Input: part model. Units: mm. Frame: model coordinates. Face numbers are marked on the shaded views. A direction names the side the tool comes from. Coordinates: 2 decimals unless noted, no trailing zeros. Write each loop counter-clockwise with the first axis right and the second up, starting at its lowest first coordinate (ties: lowest second). Pieces come first, ordered by that corner, then holes. Notation, with made-up numbers: (69, -25) - (116, -25) arc R34 ccw to (116, 7) - close; hole circle Ø3 at (51, 10.25). An arc over 180 degrees is marked (long way). Use CSV: the item, a comma, the result in double quotes.
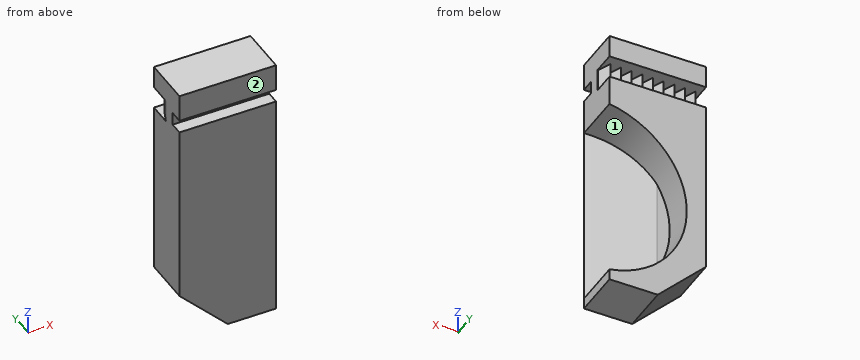
```python
from build123d import *

# Parameters (mm, degrees)
ESQUISSE2_W                = 30
ESQUISSE2_H                = 84
BOSS_EXTRU_1_DEPTH         = 15
ESQUISSE3_R                = 29
ENL_V_MAT_EXTRU_1_DEPTH    = 10
CHANFREIN1_SIZE            = 5
CHANFREIN1_SIZE_2          = 20
CHANFREIN2_SIZE            = 15
ESQUISSE7_W                = 30
ESQUISSE7_H                = 7
ENL_V_MAT_EXTRU_2_DEPTH    = 7
BOSS_EXTRU_2_DEPTH         = 7
R_P_TITION_LIN_AIRE1_COUNT = 9
R_P_TITION_LIN_AIRE1_PITCH = 3.31
ENL_V_MAT_EXTRU_3_REACH    = 56.708
ESQUISSE9_W                = 4
ESQUISSE9_H                = 4


with BuildPart() as part:
    # Esquisse2 → Boss.-Extru.1 (new body)
    with BuildSketch(Plane(origin=(0, 0, 0), x_dir=(1, 0, 0), z_dir=(0, 1, 0))):
        with Locations((-17.412854797, -1.219560319)):
            Rectangle(ESQUISSE2_W, ESQUISSE2_H)
    extrude(amount=BOSS_EXTRU_1_DEPTH)

    # Esquisse3 → Enlèv. mat.-Extru.1 (cut)
    with BuildSketch(Plane(origin=(0, 15, 0), x_dir=(1, 0, 0), z_dir=(0, 1, 0))):
        with Locations((2.587145203, 8.780439681)):
            Circle(ESQUISSE3_R)
    extrude(amount=-ENL_V_MAT_EXTRU_1_DEPTH, mode=Mode.SUBTRACT)

    # Chanfrein1
    # the kernel refuses this chamfer: 20, 5 mm, written as the material it takes off along each edge
    with BuildSketch(Plane(origin=(-2.412854797, 5, -89.288703391), x_dir=(0.14778356633657125, -0.9890197255468893, 0), z_dir=(0, 0, 1))) as chanfrein1_piece_1_section:
        Polygon((CHANFREIN1_SIZE * 0.989019725547, -CHANFREIN1_SIZE * 0.147783566337), (-CHANFREIN1_SIZE_2 * 0.147783566337, -CHANFREIN1_SIZE_2 * 0.989019725547), (0, 0), align=None)
    chanfrein1_piece_1 = extrude(amount=161.016527419, mode=Mode.PRIVATE)
    chanfrein1_piece_1 = chanfrein1_piece_1 & Plane(origin=(2.587145203, 3.276810051, -8.780439681), x_dir=(1, 0, 0), z_dir=(0, 1, 0)) * Cylinder(29, 402, mode=Mode.PRIVATE)
    add(chanfrein1_piece_1, mode=Mode.SUBTRACT)

    # Chanfrein2
    chanfrein2_edges = [part.edges().sort_by_distance(p)[0] for p in [
        (-32.412854797, 7.5, -40.780439681),
    ]]
    chamfer(chanfrein2_edges, length=CHANFREIN2_SIZE)

    # Esquisse7 → Enlèv. mat.-Extru.2 (cut)
    with BuildSketch(Plane(origin=(0, 15, 0), x_dir=(1, 0, 0), z_dir=(0, 1, 0))):
        with Locations((-17.412854797, -32.719560319)):
            Rectangle(ESQUISSE7_W, ESQUISSE7_H)
    extrude(amount=-ENL_V_MAT_EXTRU_2_DEPTH, mode=Mode.SUBTRACT)

    # Esquisse8 → Boss.-Extru.2 (add)
    with BuildSketch(Plane.XY.offset(29.219560319)):
        Polygon((-32.412854797, 8), (-29.099146298, 8), (-30.756000548, 12), align=None)
    boss_extru_2 = extrude(amount=BOSS_EXTRU_2_DEPTH)

    # Répétition linéaire1: Boss.-Extru.2 ×9
    with Locations(*[(i * R_P_TITION_LIN_AIRE1_PITCH, 0, 0) for i in range(1, R_P_TITION_LIN_AIRE1_COUNT)]):
        add(boss_extru_2)

    # Esquisse9 → Enlèv. mat.-Extru.3 (cut, up to next)
    with BuildSketch(Plane(origin=(-2.412854797, 0, 0), x_dir=(0, 0, -1), z_dir=(1, 0, 0)), mode=Mode.PRIVATE) as enl_v_mat_extru_3_sk1:
        with Locations((-32.719560319, 2)):
            Rectangle(ESQUISSE9_W, ESQUISSE9_H)
    enl_v_mat_extru_3_tool1 = extrude(enl_v_mat_extru_3_sk1.sketch, amount=-ENL_V_MAT_EXTRU_3_REACH, mode=Mode.PRIVATE) & part.part
    add(enl_v_mat_extru_3_tool1.solids().sort_by_distance((-2.412855, 2, 32.71956))[0], mode=Mode.SUBTRACT)


solid = part.part
```
(1) Ray query, probe 1 along Z at (x, y) = (-18.5, 12.5); probe 2 along Z at (x, y) = (-19, 8.75); probe 3 along Z at (x, y) = (-11, 1). Return the intervals inside material, ascending. Write a range as from..to.
Check values:
probe 1,"-39.69..-28.69, 11.13..29.22, 36.22..43.22"
probe 2,"-39.19..-28.15, 10.58..29.22, 36.22..43.22"
probe 3,"-40.78..30.72, 34.72..43.22"
(2) Cut plane C-C on x = -15. Return loops of the section in (y, z), and give its area (3 significant figures).
Check values:
outline,"(0, -40.78) - (15, -40.78) - (15, -31.84) - (3.15, -31.84) - (3.15, 14.28) - (15, 14.28) - (15, 29.22) - (10.08, 29.22) - (10.08, 36.22) - (15, 36.22) - (15, 43.22) - (0, 43.22) - (0, 34.72) - (4, 34.72) - (4, 30.72) - (0, 30.72) - close"
area,"663 mm^2"
(3) Reachability of the marked faces 1 and 2 from +Z, -Z, +X, -X, +Y, -Y: full face, straight path, thin tool, end or side. Return the list, or none.
Check values:
face 1,"+X, +Y"
face 2,"+Z, -Z, +X, -X, -Y"
(4) Pin query (flat end, axial travel): pin 1 Ø4.5 at (x, z) = (-24.5, -3.5) entering from +Y; pin 2 Ø3 at (y, z) = (6.5, -29) entering from -X. Return the tip coordinate at first contact, or that it passes through.
Check values:
pin 1,"y = 15"
pin 2,"x = -30.69"
(5) Cut plane A-A on y = 1. Return loops of the section in (x, z).
Check values:
outline,"(-32.41, -25.78) - (-17.41, -40.78) - (-2.41, -40.78) - (-2.41, -37.35) arc R29 cw to (-6.41, -36.35) - (-6.41, 18.79) arc R29 cw to (-2.41, 19.79) - (-2.41, 30.72) - (-32.41, 30.72) - close; (-32.41, 34.72) - (-2.41, 34.72) - (-2.41, 43.22) - (-32.41, 43.22) - close"
(6) Cut plane B-B on y = 7.25. Return loops of the section in (x, z), and give its area (3 significant figures).
Check values:
outline,"(-32.41, -25.78) - (-17.41, -40.78) - (-2.41, -40.78) - (-2.41, -37.35) arc R29 cw to (-2.41, 19.79) - (-2.41, 43.22) - (-32.41, 43.22) - close"
area,"1,380 mm^2"
(7) Cut plane D-D on z = 15. Return loops of the section in (x, y).
Check values:
outline,"(-32.41, 0) - (-2.41, 0) - (-14.01, 2.9) - (-14.01, 15) - (-32.41, 15) - close"
